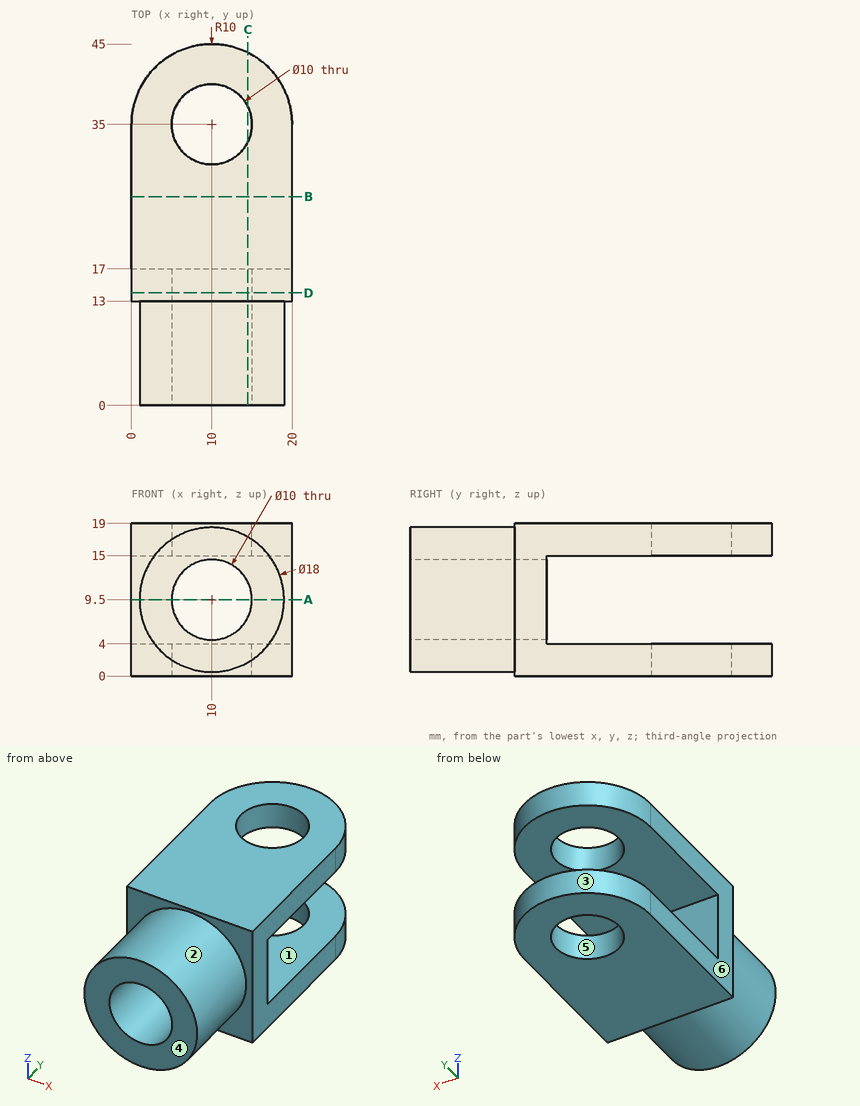
The figure shows three views and two pictorial views of one solid part (mm, origin at its lowest corner). Answer the questions. A direction names the side the tool comes from. Round coordinates to 2 decimals unless told otherwise and drop trailing zeros. Write each loop counter-clockwise with the first axis right and the second up, starting at its lowest first coordinate (ties: lowest second). Pieces come first, ordered by that corner, then holes. Notation, with made-up numbers: M 46,61 L 84,61 A31 cw 84,86 Z; hole C 56,-16 d1. An arc over 180 degrees is marked long. Use a Markdown table: item, result.
1) The part is cut by section C-C on x = 14.5. Give the vertices of the cut face in (y, z), plus the area to 3 significant figures.
Taken from the geometry:
| item | result |
|---|---|
| outline | M 0,1.71 L 13,1.71 L 13,0 L 32.82,0 L 32.82,4 L 17,4 L 17,7.32 L 0,7.32 Z; M 0,11.68 L 17,11.68 L 17,15 L 32.82,15 L 32.82,19 L 13,19 L 13,17.29 L 0,17.29 Z; M 37.18,0 L 43.93,0 L 43.93,4 L 37.18,4 Z; M 37.18,15 L 43.93,15 L 43.93,19 L 37.18,19 Z |
| area | 385 mm2 |
2) The part is cut by section B-B on y = 26. Give the vertices of the cut face in (x, z), plus the area to 3 significant figures.
Taken from the geometry:
| item | result |
|---|---|
| outline | M 0,0 L 20,0 L 20,4 L 0,4 Z; M 0,15 L 20,15 L 20,19 L 0,19 Z |
| area | 160 mm2 |
3) The part is cut by section D-D on y = 14. Give the vertices of the cut face in (x, z), plus the area to 3 significant figures.
Taken from the geometry:
| item | result |
|---|---|
| outline | M 0,0 L 20,0 L 20,19 L 0,19 Z; hole C 10,9.5 d10 |
| area | 301 mm2 |
4) Determine the mould class of the marked faces 4, 5 and 6 for opening direction Y: pulls with the +Y half, pulls with the -Y half, needs draft (parallel to the pull), parting line crosses it, or undercut.
Taken from the geometry:
| item | result |
|---|---|
| face 4 | pulls with the -Y half |
| face 5 | undercut |
| face 6 | needs draft |
5) Flat-ended cylindrical pins translate along their axes: pin 1 (8 mm diameter, centred on y = 6, z = 5.5, fed in from -X); pin 2 (3 mm diameter, centred on y = 40, z = 14.5, fed in from -X) (3 decimals). Find the tip coordinate at first contact, or state that the pin passes through.
Taken from the geometry:
| item | result |
|---|---|
| pin 1 | stops at x = 1 |
| pin 2 | stops at x = 0.665 |
6) Which of the six approach directions +Z, -Z, +X, -X, +Y, -Y give full straight-line access (tool end or side, diameter ignored) to the marked faces 1, 2 and 3?
Taken from the geometry:
| item | result |
|---|---|
| face 1 | +X, -X, +Y |
| face 2 | -Y |
| face 3 | +Z, -Z, +Y |
7) Consider line 1 (Z direction, x = 9, y = 23.5); line 2 (Y direction, x = 10, z = 1.35); line 3 (X direction, y = 35, z = 1.2). Determine where each line is inside the solid, lowest interval first. Write a range as [from, to].
Taken from the geometry:
| item | result |
|---|---|
| line 1 | z = [0, 4], [15, 19] |
| line 2 | y = [0, 30], [40, 45] |
| line 3 | x = [0, 5], [15, 20] |
8) The part is cut by section A-A on z = 9.5. Give the vertices of the cut face in (x, y).
Taken from the geometry:
| item | result |
|---|---|
| outline | M 0,13 L 1,13 L 1,0 L 5,0 L 5,17 L 0,17 Z; M 15,0 L 19,0 L 19,13 L 20,13 L 20,17 L 15,17 Z |
